Can you work these out from the drawing? Everything is in mm from the part's minimum corner. A direction names the side the tool comes from. Round coordinates to 2 decimals unless told otherwise and drop trailing zeros. Write each loop counter-clockwise with the first axis right and the second up, starting at its lowest first coordinate (ties: lowest second). Pieces come first, ordered by that corner, then holes.
Q1. I'm going to push a flat-ended pin straight in: pin 1 Ø5 at (x, z) = (6, 5.5) entering from +Y. Where does the tip first touch, or does it pass through?
Q2. If we section it at B-B (z = 9.25): Please give me the cut outline in (x, y).
Q3. We'd pull the mould along X, two halves only. Please class the marked faces 3, 4 and 5: +X half, -X half, draft (parallel to the pull), parting line (faces both ways), or undercut.
Q4. If we section it at A-A (x = 6): Please give me the cut outline in (y, z).
Q5. If we section it at C-C (y = 1): Give the number of separate pieces and of enclosed holes in the cut face, plus the area to 3 significant figures.
Q6. If we section it at D-D (x = 16.75): Please give me the cut outline in (y, z).
Q7. For the marked faces 1 and 2, which set-ups out of +Z, -Z, +X, -X, +Y, -Y let a thin tool reach every point of the face, with its end or its side?
Q8. Please list where these lines run through material, in increasing order: line 1 along X through (y, z) = (3.6, 16.75); line 2 along X through (y, z) = (0.45, 21.5).
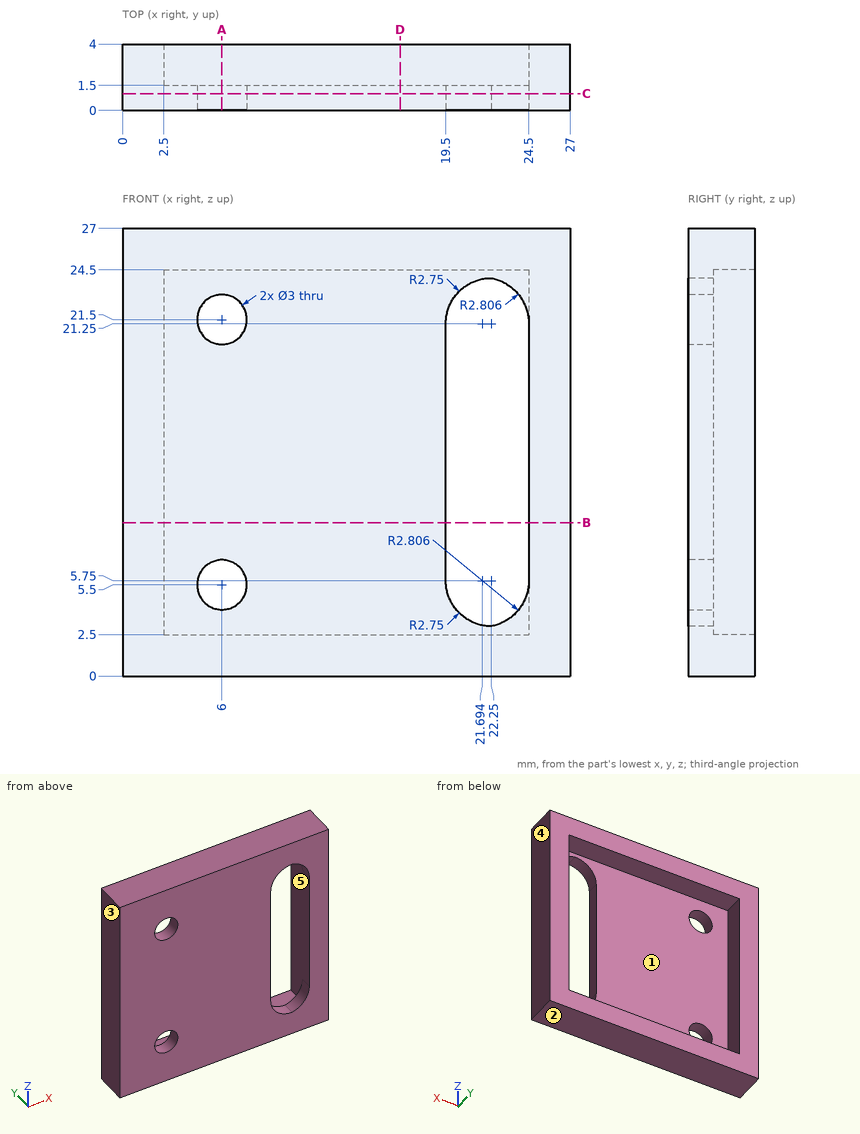
A:
1. pin 1: stops at y = 1.5
2. outline: (0, 0) - (19.5, 0) - (19.5, 1.5) - (2.5, 1.5) - (2.5, 4) - (0, 4) - close; (24.5, 0) - (27, 0) - (27, 4) - (24.5, 4) - close
3. face 3: -X half
3. face 4: +X half
3. face 5: undercut
4. outline: (0, 0) - (4, 0) - (4, 2.5) - (1.5, 2.5) - (1.5, 4) - (0, 4) - close; (0, 7) - (1.5, 7) - (1.5, 20) - (0, 20) - close; (0, 23) - (1.5, 23) - (1.5, 24.5) - (4, 24.5) - (4, 27) - (0, 27) - close
5. separate pieces: 1
5. enclosed holes: 3
5. area: 616 mm2
6. outline: (0, 0) - (4, 0) - (4, 2.5) - (1.5, 2.5) - (1.5, 24.5) - (4, 24.5) - (4, 27) - (0, 27) - close
7. face 1: +Y
7. face 2: -Z, +X, -X, +Y, -Y
8. line 1: x = 0 to 2.5, 24.5 to 27
8. line 2: x = 0 to 4.5, 7.5 to 19.51, 24.49 to 27
